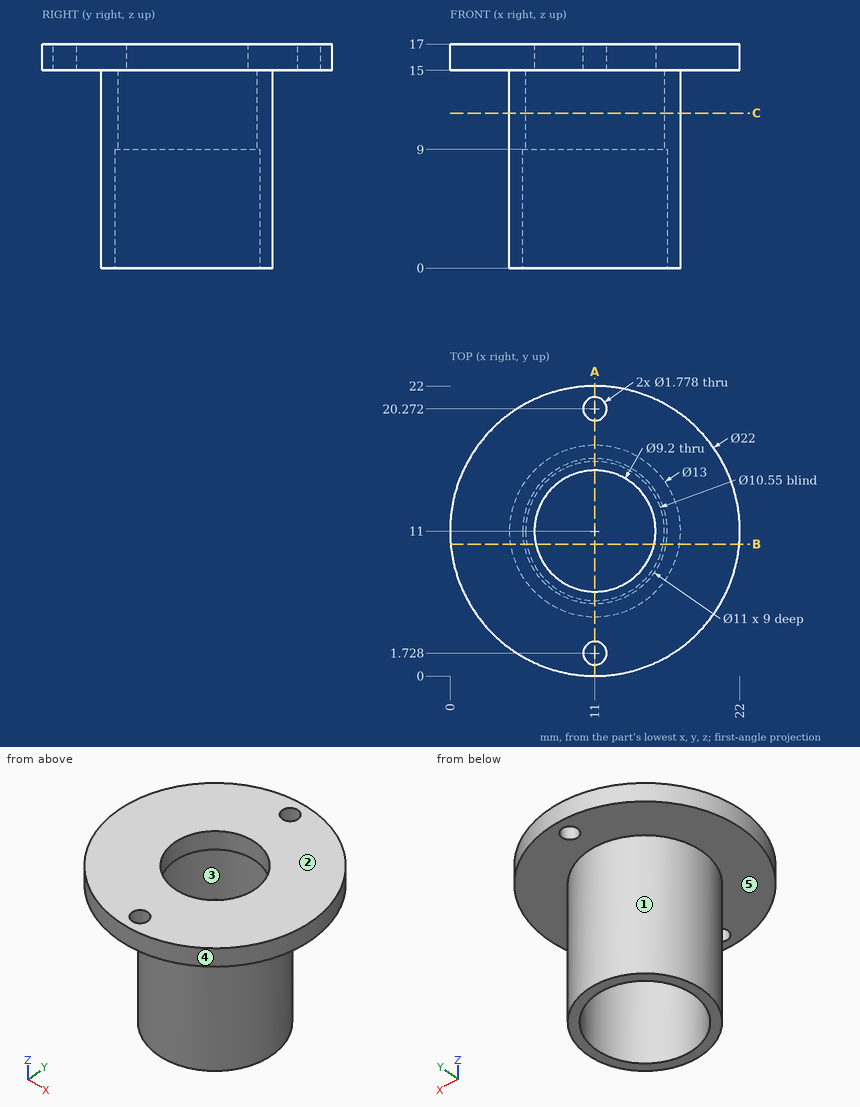
Input: dimensioned drawing with shaded views. Units: mm. Origin: part minimum x, y, z. A direction names the side the tool comes from. Round coordinates to 2 decimals unless told otherwise and drop trailing zeros. Loops run counter-clockwise (first coordinate to the right, second up) from the corner with the lowest first, then second, coordinate; pieces in that order, holes last. Notation, with made-up numbers: M 15.5,52.5 L 59.5,52.5 A7 ccw 59.5,59.5 Z; hole C 47.5,-7 d8. An arc over 180 degrees is marked long. Answer in a Markdown table with one row per item. Add a question column.
1. Section C-C (z = 11.75). Output: boundary loops of the cut face in (x, y) (3 decimals), and give its area (3 significant figures).
2. Ray query, probe 1 along Y at (x, z) = (11, 15.8); probe 2 along Y at (x, z) = (11, 14) (3 decimals). Return the intervals inside material, ascending.
3. Set-up query: the marked faces 1 and 2. Return all of +Z, -Z, +X, -X, +Y, -Y with unobstructed straight access to the full face (end or side cutting, diameter ignored); none if empty.
4. Section A-A (x = 11). Give the number of separate pieces and of enclosed holes in the cut face, and give its area (3 significant figures).
5. Mould query, pull axis X, two halves, no side actions, for the marked faces 3, 4 and 5. Classes: released by +X, released by -X, zero draft, split by the parting line, or undercut.
6. Contact query for flat-ended pins moving along their axis: pin 1 (1.1 mm diameter, centred on x = 11, y = 20.27, fed in from -Z); pin 2 (4 mm diameter, centred on x = 19, z = 8.5, fed in from -Y); pin 3 (3 mm diameter, centred on x = 16, y = 18.5, fed in from -Z); pin 4 (8 mm diameter, centred on x = 6.5, z = 10, fed in from -Y). Output: stop coordinate, or through.
7. Section B-B (y = 10). Output: boundary loops of the cut face in (x, z).
Values follow:
| question | item | result |
|---|---|---|
| 1 | outline | C 11,11 d13; hole C 11,11 d10.55 |
| 1 | area | 45.3 mm^2 |
| 2 | probe 1 | 0 to 0.84, 2.62 to 6.4, 15.6 to 19.38, 21.16 to 22 |
| 2 | probe 2 | 4.5 to 5.725, 16.275 to 17.5 |
| 3 | face 1 | -Z |
| 3 | face 2 | +Z, +X, -X, +Y, -Y |
| 4 | separate pieces | 4 |
| 4 | enclosed holes | 0 |
| 4 | area | 51.2 mm^2 |
| 5 | face 3 | undercut |
| 5 | face 4 | split by the parting line |
| 5 | face 5 | zero draft |
| 6 | pin 1 | through |
| 6 | pin 2 | y = 8.5 |
| 6 | pin 3 | z = 15 |
| 6 | pin 4 | y = 4.52 |
| 7 | outline | M 0.05,15 L 4.58,15 L 4.58,0 L 5.59,0 L 5.59,9 L 5.82,9 L 5.82,15 L 6.51,15 L 6.51,17 L 0.05,17 Z; M 15.49,15 L 16.18,15 L 16.18,9 L 16.41,9 L 16.41,0 L 17.42,0 L 17.42,15 L 21.95,15 L 21.95,17 L 15.49,17 Z |
